from build123d import *

# Parameters (mm, degrees)
SKETCH1_W                = 180
SKETCH1_H                = 99
BOSS_EXTRUDE1_DEPTH      = 6
F_4_0_4_DIAMETER_HOLE1_D = 4
F_4_0_4_DIAMETER_HOLE2_D = 4
LPATTERN1_COUNT          = 2
LPATTERN1_PITCH          = 97
LPATTERN2_COUNT          = 2
LPATTERN2_PITCH          = 81
CHAMFER1_SIZE            = 0.8


with BuildPart() as part:
    # Sketch1 → Boss-Extrude1 (new body)
    with BuildSketch(Plane(origin=(0, 0, 0), x_dir=(1, 0, 0), z_dir=(0, 1, 0))):
        with Locations((27.155172414, -14.50862069)):
            Rectangle(SKETCH1_W, SKETCH1_H)
    extrude(amount=BOSS_EXTRUDE1_DEPTH)

    # Ø4.0 (4) Diameter Hole1 (through all)
    with Locations(Plane(origin=(0, 6, 0), x_dir=(1, 0, 0), z_dir=(0, 1, 0))):
        with Locations((111.155172414, -59.00862069)):
            f_4_0_4_diameter_hole1 = Hole(F_4_0_4_DIAMETER_HOLE1_D / 2)

    # Ø4.0 (4) Diameter Hole2 (through all)
    with Locations(Plane(origin=(0, 6, 0), x_dir=(1, 0, 0), z_dir=(0, 1, 0))):
        with Locations((55.155172414, 29.99137931)):
            f_4_0_4_diameter_hole2 = Hole(F_4_0_4_DIAMETER_HOLE2_D / 2)

    # LPattern1: Ø4.0 (4) Diameter Hole1 ×2
    with Locations(*[(-i * LPATTERN1_PITCH, 0, 0) for i in range(1, LPATTERN1_COUNT)]):
        add(f_4_0_4_diameter_hole1, mode=Mode.SUBTRACT)

    # LPattern2: Ø4.0 (4) Diameter Hole2 ×2
    with Locations(*[(-i * LPATTERN2_PITCH, 0, 0) for i in range(1, LPATTERN2_COUNT)]):
        add(f_4_0_4_diameter_hole2, mode=Mode.SUBTRACT)

    # Chamfer1
    chamfer1_edges = [part.edges().sort_by_distance(p)[0] for p in [
        (117.155172414, 6, 14.50862069),
        (27.155172414, 6, -34.99137931),
        (-62.844827586, 6, 14.50862069),
        (27.155172414, 6, 64.00862069),
    ]]
    chamfer(chamfer1_edges, length=CHAMFER1_SIZE)


solid = part.part
Verification items for the finished model (mm, model axes). Round coordinates to 2 decimals unless told otherwise and drop trailing zeros. Use a Markdown table: item, result. Add a question column.
1. Gauge pin test, flat end, axial feed: pin 1 (3 mm diameter, centred on x = -25.84, z = -29.99, fed in from +Y). Record the tip position at first contact, or that the pin passes through.
2. Release check for a two-part mould opening along Z. For faces 1 (the face through (54.08, 2.96, -31.68)), 2 (the face through (26, 3, 64.009)), 3 (the face through (111.59, 2.96, 60.96)), 4 (the face through (-62.845, 3, 15)) record: released by +Z, released by -Z, zero draft, split by the parting line, or undercut.
3. Thickness scan on probe 1 along X at (y, z) = (0.4, -30); probe 2 along X at (y, z) = (0.65, 59.5). Record the ranges inside material, lowest first. Write a range as [from, to].
Checks:
| question | item | result |
|---|---|---|
| 1 | pin 1 | passes through |
| 2 | face 1 | undercut |
| 2 | face 2 | released by +Z |
| 2 | face 3 | undercut |
| 2 | face 4 | zero draft |
| 3 | probe 1 | x = [-62.84, -27.84], [-23.84, 53.16], [57.16, 117.16] |
| 3 | probe 2 | x = [-62.84, 12.22], [16.09, 109.22], [113.09, 117.16] |
